Can you work these out from the model? Positions are in its coordinate system, mm. A direction names the side the tool comes from. Coordinates: 2 decimals unless noted, no trailing zeros. Order: outer loops, then holes, each group sorted by start corner. A loop starts at its lowest first (then second) coordinate and runs counter-clockwise, first axis right, second up. Notation, with made-up numbers: (55, -23.5) -> (64, -23.5) arc R19 ccw to (64, 10.5) -> close; hole circle Ø11 at (-35, 35). An arc over 180 degrees is marked (long way). Answer in a Markdown table with one row per item.
Autodesk Inventor part; units mm, degrees
ref_plane "YZ Plane" through (0, 0, 0) normal (1, 0, 0) x (0, 1, 0)
ref_plane "XZ Plane" through (0, 0, 0) normal (0, 1, 0) x (-1, 0, 0)
ref_plane "XY Plane" through (0, 0, 0) normal (0, 0, 1) x (1, 0, 0)
sketch "Sketch1" plane through (0, 0, 0) normal (0, 0, 1) x (1, 0, 0)
  line L0 (5.6515, 0) -> (36.6485, 0)
  line L1 (42.3, 5.6515) -> (42.3, 36.6485)
  line L2 (36.6485, 42.3) -> (5.6515, 42.3)
  line L3 (0, 36.6485) -> (0, 5.6515)
  line L4 (0, 36.6485) -> (5.6515, 42.3)
  line L5 (36.6485, 42.3) -> (42.3, 36.6485)
  line L6 (42.3, 5.6515) -> (36.6485, 0)
  line L7 (5.6515, 0) -> (0, 5.6515)
  line L8 (21.15, 42.3) -> (21.15, 0) construction
  line L9 (0, 21.9578) -> (42.3, 21.9578) construction
  point P0 (0, 0)
  point P1 (42.3, 42.3)
  point P2 (42.3, 0)
  point P3 (0, 42.3)
  dimension "d0" = 42.3
  dimension "d1" = 42.3
  dimension "d2" = 5.6515
  dimension "d3" = 5.6515
  dimension "d4" = 5.6515
  dimension "d5" = 5.6515
  dimension "d6" = 5.6515
  dimension "d7" = 5.6515
  dimension "d8" = 5.6515
  dimension "d9" = 5.6515
  dimension "d10" = 30.997
extrude "Extrusion1" add sketch "Sketch1" along normal blind 33.02
sketch "Sketch2" plane through (0, 0, 33.02) normal (0, 0, 1) x (1, 0, 0)
  line L0 (5.6515, 42.3) -> (36.6485, 42.3)
  line L1 (0, 5.6515) -> (0, 36.6485)
  line L2 (36.6485, 0) -> (5.6515, 0)
  line L3 (42.3, 36.6485) -> (42.3, 5.6515)
  line L4 (21.15, 42.3) -> (21.15, 0) construction
  line L5 (0, 21.15) -> (42.3, 21.15) construction
  circle A0 centre (21.15, 21.15) radius 11
  point P0 (0, 0)
  dimension "d13" = 22
extrude "Extrusion2" add sketch "Sketch2" along normal blind 2
sketch "Sketch3" plane through (21.15, 21.15, 35.02) normal (0, 0, 1) x (1, 0, 0)
  circle A0 centre (0, 0) radius 11
  arc A1 (0, 2.5) -> (1.4504, -2.0363) centre (0, 0) ccw
  line L0 (0, 2.5) -> (1.4504, -2.0363)
  point P0 (-21.15, -21.15)
  dimension "d16" = 5
  dimension "d17" = 4.7625
extrude "Extrusion3" add sketch "Sketch3" along normal blind 16.002 contours L0 A1
sketch "Sketch4" plane through (0, 0, 33.02) normal (0, 0, 1) x (1, 0, 0)
  line L0 (0, 36.6485) -> (5.6515, 42.3)
  line L1 (5.6515, 0) -> (0, 5.6515)
  line L2 (42.3, 5.6515) -> (36.6485, 0)
  line L3 (36.6485, 42.3) -> (42.3, 36.6485)
  line L4 (2.8258, 39.4742) -> (39.4742, 2.8258) construction
  line L5 (39.4742, 39.4742) -> (2.8257, 2.8258) construction
  point P0 (0, 0)
  point P1 (5.65, 36.65)
  point P2 (36.65, 36.65)
  point P3 (5.65, 5.65)
  point P4 (36.65, 5.65)
  dimension "d20" = 31
  dimension "d21" = 31
  dimension "d22" = 31
  dimension "d23" = 31
hole "Hole1" at (5.65, 36.65, 33.02) at (36.65, 36.65, 33.02) at (5.65, 5.65, 33.02) at (36.65, 5.65, 33.02) direction (0, 0, -1) diameter 4 end through all
properties part number "stepper42BYGH007" material "Aluminum-6061"
(1) Suppose I cut it at B-B (y = 36). Please give me the cut outline in (x, z), and give its area (3 significant figures).
Response values:
| item | result |
|---|---|
| outline | (0, 0) -> (3.76, 0) -> (3.76, 33.02) -> (0, 33.02) -> close; (7.54, 0) -> (34.76, 0) -> (34.76, 33.02) -> (7.54, 33.02) -> close; (38.54, 0) -> (42.3, 0) -> (42.3, 33.02) -> (38.54, 33.02) -> close |
| area | 1,150 mm2 |
(2) Suppose I cut it at D-D (y = 16). Please give me the cut outline in (x, z), and give its area (3 significant figures).
Response values:
| item | result |
|---|---|
| outline | (0, 0) -> (42.3, 0) -> (42.3, 33.02) -> (30.87, 33.02) -> (30.87, 35.02) -> (11.43, 35.02) -> (11.43, 33.02) -> (0, 33.02) -> close |
| area | 1,440 mm2 |
(3) On a 3-axis mill with a long thin cutter (end or side, diameter ignored), from which of +Z, -Z, +X, -X, +Y, -Y can I reach the whole of each face in a straight line? I mean faces 4 (the cylindrical face through (10.16, 20.67, 34.01)), 5 (the cylindrical face through (37.416, 34.803, 16.279)), 6 (the flat face through (21.865, 21.414, 42.909)). Say none if no direction works.
Response values:
| item | result |
|---|---|
| face 4 | +Z |
| face 5 | +Z, -Z |
| face 6 | +Z, +X, +Y |
(4) We'd pull the mould along X, two halves only. Please class faces 1 (the flat face through (23, 21, 35.02)), 2 (the cylindrical face through (6.416, 34.803, 16.279)), 3 (the flat face through (0, 21, 16)): +X half, -X half, draft (parallel to the pull), parting line (faces both ways), or undercut.
Response values:
| item | result |
|---|---|
| face 1 | draft |
| face 2 | undercut |
| face 3 | -X half |
(5) Suppose I cut it at A-A (z = 24.5). Please give me the cut outline in (x, y).
Response values:
| item | result |
|---|---|
| outline | (0, 5.65) -> (5.65, 0) -> (36.65, 0) -> (42.3, 5.65) -> (42.3, 36.65) -> (36.65, 42.3) -> (5.65, 42.3) -> (0, 36.65) -> close; hole circle Ø4 at (5.65, 5.65); hole circle Ø4 at (5.65, 36.65); hole circle Ø4 at (36.65, 5.65); hole circle Ø4 at (36.65, 36.65) |
(6) I need wall thicknesses on line 1 (Y direction, x = 36.65, z = 15.5); line 2 (Y direction, x = 36, z = 11); line 3 (X direction, y = 7, z = 16). Which ranges of each line are inside material? Lowest first, please. Write a range as [from, to].
Response values:
| item | result |
|---|---|
| line 1 | [0, 3.65], [7.65, 34.65], [38.65, 42.3] |
| line 2 | [0, 3.76], [7.54, 34.76], [38.54, 42.3] |
| line 3 | [0, 4.17], [7.13, 35.17], [38.13, 42.3] |
(7) Will this pin go through, and if not, where does the flat tip stop? pin 1 Ø1 at (x, y) = (7, 19) entering from +Z.
Response values:
| item | result |
|---|---|
| pin 1 | z = 33.02 |
(8) Suppose I cut it at C-C (x = 25.5). Please give me the cut outline in (y, z).
Response values:
| item | result |
|---|---|
| outline | (0, 0) -> (42.3, 0) -> (42.3, 33.02) -> (31.25, 33.02) -> (31.25, 35.02) -> (11.05, 35.02) -> (11.05, 33.02) -> (0, 33.02) -> close |
